Check sheet for the drawn part. Datum: minimum x, y, z corner. Units: mm. Round coordinates to 2 decimals unless told otherwise and drop trailing zeros. Order: outer loops, then holes, each group sorted by start corner. A loop starts at its lowest first (then second) coordinate and runs counter-clockwise, first axis right, second up. Notation, with made-up numbers: M 8.5,89.25 L 57.5,89.25 A18 cw 57.5,120.25 Z; hole C 36,64.5 d4. An arc over 180 degrees is marked long. Write item = value, one per line. Start each with the question number.
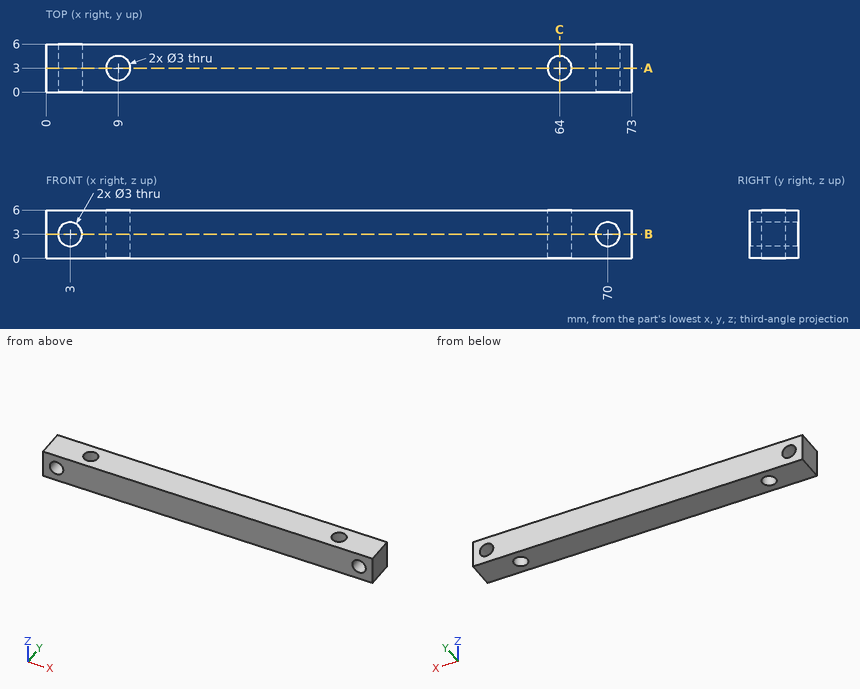
1) Cross-section at A-A, the plane y = 3. Enter the section's corners in (x, z).
2) Scan lines: probe 1 along Z at (x, y) = (3, 4.5); probe 2 along X at (y, z) = (3, 3.4). Record each from-to range of solid material in increasing order.
3) Gauge pin test, flat end, axial feed: P1, Ø2.5, axis at x = 3, z = 3, coming from the -Y side. Record the tip position at first contact, or that the pin passes through.
4) Cross-section at B-B, the plane z = 3. Enter the section's corners in (x, y), then the cut area to 3 significant figures.
5) Cross-section at C-C, the plane x = 64. Enter the section's corners in (y, z).
Geometry results:
q1.outline = M 0,0 L 7.5,0 L 7.5,6 L 0,6 Z; M 10.5,0 L 62.5,0 L 62.5,6 L 10.5,6 Z; M 65.5,0 L 73,0 L 73,6 L 65.5,6 Z; hole C 3,3 d3; hole C 70,3 d3
q2.probe_1 = 0 to 1.5, 4.5 to 6
q2.probe_2 = 0 to 1.55, 4.45 to 7.5, 10.5 to 62.5, 65.5 to 68.55, 71.45 to 73
q3.P1 = through
q4.outline = M 0,0 L 1.5,0 L 1.5,6 L 0,6 Z; M 4.5,0 L 68.5,0 L 68.5,6 L 4.5,6 Z; M 71.5,0 L 73,0 L 73,6 L 71.5,6 Z; hole C 9,3 d3; hole C 64,3 d3
q4.area = 388 mm^2
q5.outline = M 0,0 L 1.5,0 L 1.5,6 L 0,6 Z; M 4.5,0 L 6,0 L 6,6 L 4.5,6 Z
